from build123d import *

# Parameters (mm, degrees)
F0_R     = 8
F0_R_2   = 5
F1_DEPTH = 50
F2_DEPTH = 2
F3_R     = 2
F4_DEPTH = 25


with BuildPart() as f1:
    # F0 (on Top) → F1 (new body)
    with BuildSketch(Plane.XY):
        Circle(F0_R)
        Circle(F0_R_2, mode=Mode.SUBTRACT)
    extrude(amount=F1_DEPTH)

    # F0 (on Top) → F2 (join)
    with BuildSketch(Plane.XY):
        Circle(F0_R_2)
    extrude(amount=F2_DEPTH)

    # F3 (on Right) → F4 (cut)
    with BuildSketch(Plane.YZ):
        with Locations((0, 40)):
            Circle(F3_R)
    extrude(amount=-F4_DEPTH, mode=Mode.SUBTRACT)


solid = f1.part
Verification items for the finished model (mm, model axes). A direction names the side the tool comes from. Round coordinates to 2 decimals unless told otherwise and drop trailing zeros. Loops run counter-clockwise (first coordinate to the right, second up) from the corner with the lowest first, then second, coordinate; pieces in that order, holes last. Notation, with made-up numbers: (79.25, 85) - (106.25, 85) arc R36 ccw to (106.25, 121) - close; hole circle Ø10 at (-38, 23). An arc over 180 degrees is marked (long way). Use a Markdown table: item, result. Add a question column.
1. Section check D-D, the plane y = -3. Record the boundary of the cut face in (x, z), plus the area to 3 significant figures.
2. Release check for a two-part mould opening along Y. For faces 1 (the face through (0, 0, 0)), 2 (the face through (-6.3, -1.6, 38.8)), 3 (the face through (7.39, -3.06, 24.65)) record: released by +Y, released by -Y, zero draft, split by the parting line, or undercut.
3. Gauge pin test, flat ends, axial feed: pin 1 (5 mm diameter, centred on y = -2.5, z = 19, fed in from +X); pin 2 (8 mm diameter, centred on y = -5, z = 36, fed in from -X); pin 3 (3 mm diameter, centred on y = 0, z = 40, fed in from -X); pin 4 (5 mm diameter, centred on y = 5.5, z = 10.5, fed in from +X). Record the tip position at first contact, or that the pin passes through.
4. Section check B-B, the plane x = 0. Record the boundary of the cut face in (y, z).
5. Section check C-C, the plane z = 9.5. Record the boundary of the cut face in (x, y), plus the area to 3 significant figures.
6. Access from +Z, -Z, +X, -X, +Y, -Y to the whole of each face (thin tool, end or side, straight path). Record for faces 4 (the face through (0, 0, 2)), 5 (the face through (5.2, 0.1, 50)).
7. Section check A-A, the plane y = 0. Record the boundary of the cut face in (x, z), plus the area to 3 significant figures.
8. Thickness scan on probe 1 along X at (y, z) = (0, 30); probe 2 along Z at (x, y) = (-0.75, 3); probe 3 along X at (y, z) = (-3, 12). Record the ranges inside material, lowest first. Write a range as [from, to].
Checks:
| question | item | result |
|---|---|---|
| 1 | outline | (-7.42, 0) - (7.42, 0) - (7.42, 50) - (4, 50) - (4, 2) - (-4, 2) - (-4, 50) - (-7.42, 50) - close |
| 1 | area | 358 mm^2 |
| 2 | face 1 | zero draft |
| 2 | face 2 | undercut |
| 2 | face 3 | split by the parting line |
| 3 | pin 1 | stops at x = 8 |
| 3 | pin 2 | stops at x = -7.94 |
| 3 | pin 3 | stops at x = 4.77 |
| 3 | pin 4 | stops at x = 7.42 |
| 4 | outline | (-8, 0) - (8, 0) - (8, 50) - (5, 50) - (5, 2) - (-5, 2) - (-5, 50) - (-8, 50) - close |
| 5 | outline | circle Ø16 at (0, 0); hole circle Ø10 at (0, 0) |
| 5 | area | 123 mm^2 |
| 6 | face 4 | +Z |
| 6 | face 5 | +Z, +X, -X, +Y, -Y |
| 7 | outline | (-8, 0) - (8, 0) - (8, 50) - (5, 50) - (5, 2) - (-5, 2) - (-5, 38) - (-8, 38) - close; (-8, 42) - (-5, 42) - (-5, 50) - (-8, 50) - close |
| 7 | area | 308 mm^2 |
| 8 | probe 1 | x = [-8, -5], [5, 8] |
| 8 | probe 2 | z = [0, 2] |
| 8 | probe 3 | x = [-7.42, -4], [4, 7.42] |
